Geometry: see drawing. Coordinates: mm, zero at the bounding-box minimum. A direction names the side the tool comes from. Give positions to 0.01 mm unless a question says otherwise; leave off trailing zeros. Write each loop counter-clockwise with the first axis right and the second up, starting at its lowest first coordinate (ties: lowest second). Pieces come first, ordered by that corner, then holes. Notation, with made-up numbers: (-35.75, 13) - (-16.75, 13) arc R11 cw to (-16.75, 24) - close; hole circle Ø1 at (71, 0). An arc over 180 degrees is marked (long way). Use CSV: the item, a comma, the result in double quotes. Start each with the question number.
(1) Section A-A on z = 34. Output: boundary loops of the cut face in (x, y).
(2) Section C-C on y = 31. Output: boundary loops of the cut face in (x, z) (1 decimal).
(3) First-contact query: pin 1 Ø1.7 at (y, z) = (24, 90) entering from -X; pin 2 Ø1.3 at (x, z) = (26, 90) entering from -Y; pin 3 Ø1.6 at (x, z) = (18, 60.5) entering from +Y. Flat tips, straight axial feed; report the tip coordinate or a pass-through.
(4) Reachability of the marked faces 1, 2 and 3 from +Z, -Z, +X, -X, +Y, -Y: full face, straight path, thin tool, end or side. Return the list, or none.
(5) Draft query along Z for the marked faces 4, 5 and 6. Return one class per face: released by +Z, released by -Z, zero draft, split by the parting line, or undercut.
(6) Section B-B on x = 68. Count the separate pieces of the cut face and the enclosed holes in it.
(7) Line query: probe 1 along Z at (x, y) = (39.5, 13) (1 decimal); probe 2 along Y at (x, z) = (20, 12); probe 3 along Y at (x, z) = (29.5, 75). Output: solid intervals per line, ascending. Write a range as [from, to].
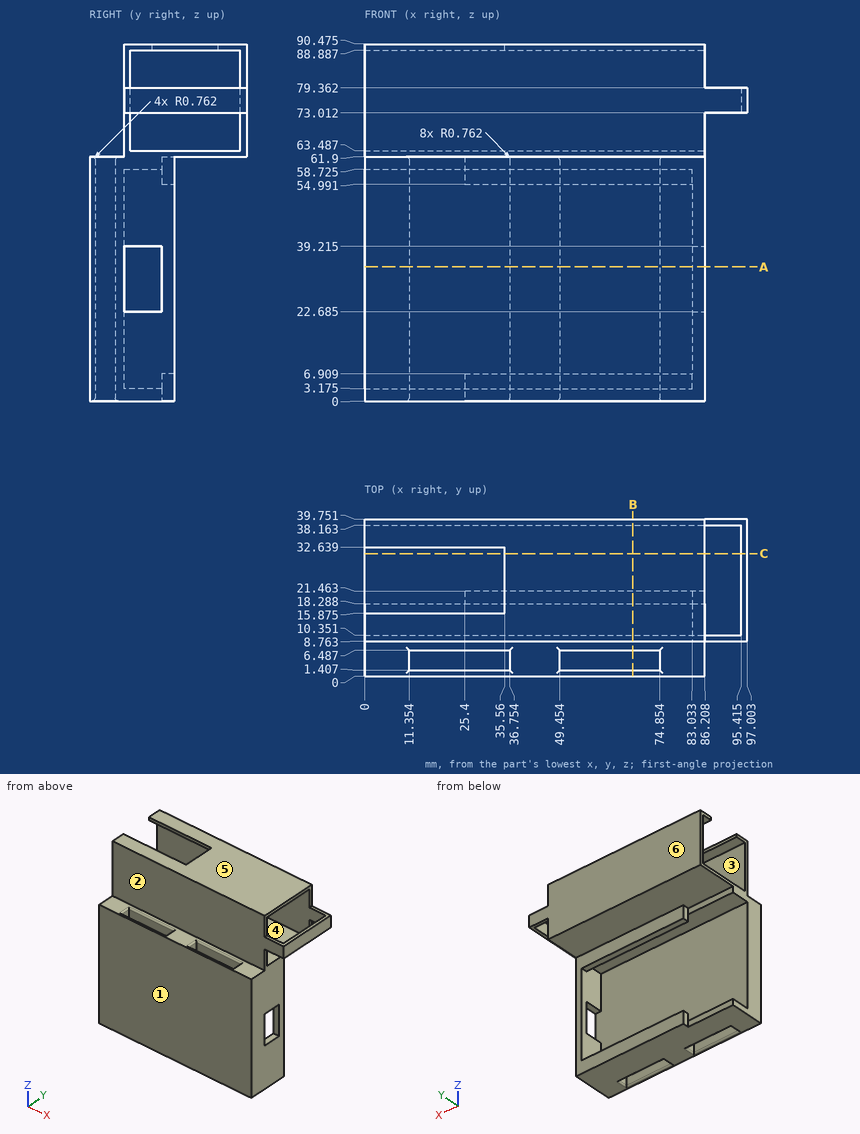
Check values:
1,outline,"(0, 0) - (86.21, 0) - (86.21, 8.76) - (0, 8.76) - close; (83.03, 18.29) - (86.21, 18.29) - (86.21, 21.46) - (83.03, 21.46) - close; hole (11.35, 1.41) - (36.75, 1.41) - (36.75, 6.49) - (11.35, 6.49) - close; hole (49.45, 1.41) - (74.85, 1.41) - (74.85, 6.49) - (49.45, 6.49) - close"
2,outline,"(0, 61.9) - (86.2, 61.9) - (86.2, 63.5) - (0, 63.5) - close; (35.6, 88.9) - (86.2, 88.9) - (86.2, 90.5) - (35.6, 90.5) - close; (95.4, 73) - (97, 73) - (97, 79.4) - (95.4, 79.4) - close"
3,pin 1,"stops at x = 35.56"
3,pin 2,"stops at y = 8.76"
3,pin 3,"stops at y = 18.29"
4,face 1,"+Z, -Z, +X, -X, -Y"
4,face 2,"+Z, +X, -X, -Y"
4,face 3,"-X"
5,face 4,"undercut"
5,face 5,"released by +Z"
5,face 6,"zero draft"
6,separate pieces,"2"
6,enclosed holes,"1"
7,probe 1,"z = [0, 3.2], [58.7, 63.5], [88.9, 90.5]"
7,probe 2,"y = [0, 1.41], [6.49, 8.76]"
7,probe 3,"y = [8.76, 10.35], [38.16, 39.75]"
